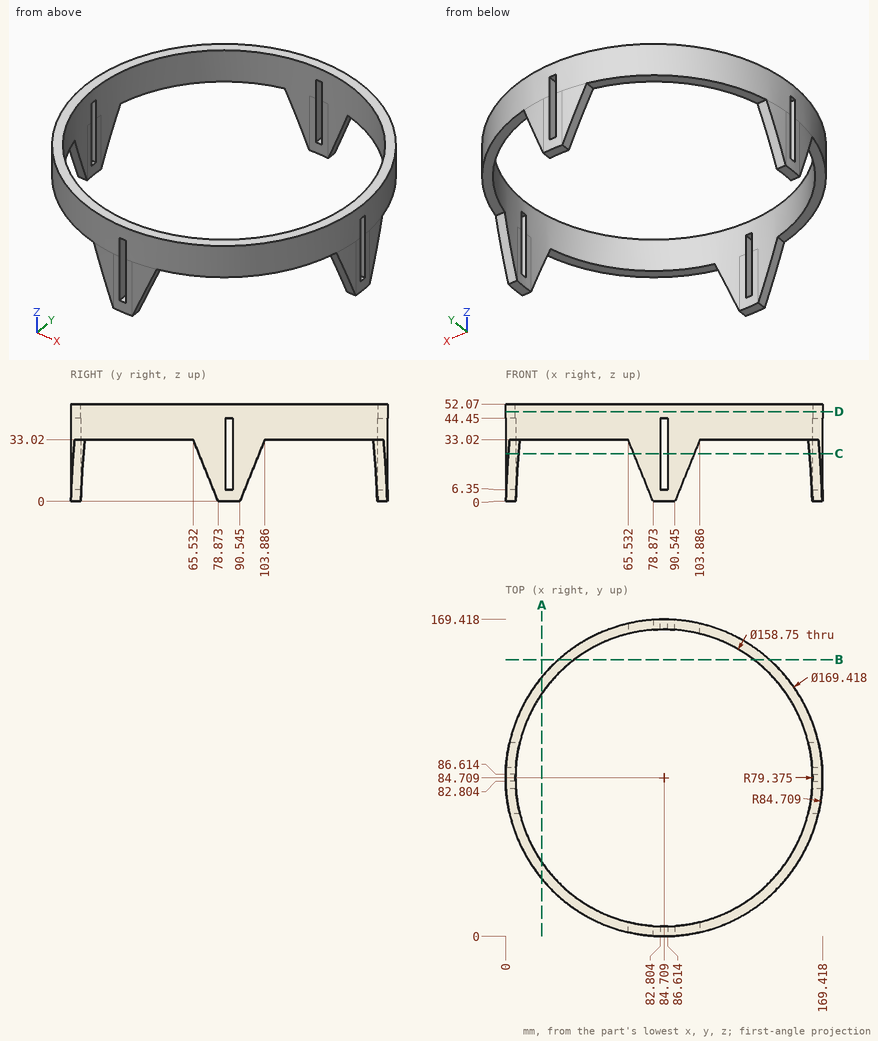
Geometry check sheet. Reference: drawing and pictorial views, mm from the part's lowest x, y, z. Coordinates: 2 decimals unless noted, no trailing zeros. Order: outer loops, then holes, each group sorted by start corner. A loop starts at its lowest first (then second) coordinate and runs counter-clockwise, first axis right, second up.
Item 1: Section check C-C, the plane z = 25.5. Give the number of separate pieces and of enclosed holes in the cut face, then the cut area to 3 significant figures.
Filled in:
separate pieces: 8
enclosed holes: 0
area: 612 mm2
Item 2: Section check D-D, the plane z = 48. Enter the section's corners in (x, y) (3 decimals).
Filled in:
outline: circle Ø169.418 at (84.709, 84.709); hole circle Ø158.75 at (84.709, 84.709)
Item 3: Section check A-A, the plane x = 19.5. Enter the section's corners in (y, z), then the cut area to 3 significant figures.
Filled in:
outline: (30.64, 33.02) - (39.45, 33.02) - (39.45, 52.07) - (30.64, 52.07) - close; (129.97, 33.02) - (138.78, 33.02) - (138.78, 52.07) - (129.97, 52.07) - close
area: 336 mm2
Item 4: Section check B-B, the plane y = 148. Enter the section's corners in (x, z).
Filled in:
outline: (28.41, 33.02) - (36.81, 33.02) - (36.81, 52.07) - (28.41, 52.07) - close; (132.61, 33.02) - (141.01, 33.02) - (141.01, 52.07) - (132.61, 52.07) - close
Item 5: Depth check by flat-ended pin: pin 1 (4.5 mm diameter, centred on y = 167, z = 29, fed in from +X); pin 2 (1.6 mm diameter, centred on y = 2, z = 28, fed in from +X); pin 3 (19 mm diameter, centred on x = 47.5, y = 18.5, fed in from -Z). Enter the tip coordinate at first touch or a pass-through.
Filled in:
pin 1: stops at x = 103.17
pin 2: stops at x = 102.18
pin 3: stops at z = 33.02
Item 6: Material ranges on L1, parallel to Y at x = 78.5, z = 27; L2, parallel to X at y = 91, z = 49; L3, parallel to X at y = 23.5, z = 44.5 (1 decimal), recorded low to high.
Filled in:
L1: y = 0.23 to 5.58, 163.84 to 169.19
L2: x = 0.23 to 5.58, 163.83 to 169.18
L3: x = 26.2 to 34.2, 135.2 to 143.3
